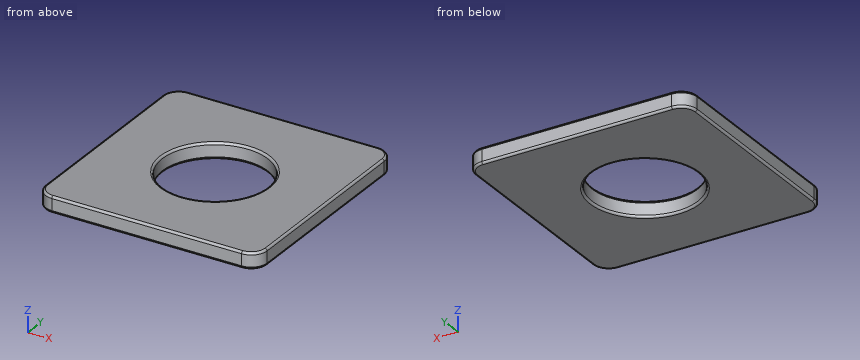
```python
from build123d import *

# Parameters (mm, degrees)
SKETCH1_W           = 21
SKETCH1_H           = 21
BOSS_EXTRUDE1_DEPTH = 0.75
FILLET1_R           = 1.5
SKETCH2_R           = 5
CUT_EXTRUDE1_DEPTH  = 15.924811557
FILLET2_R           = 0.2


with BuildPart() as part:
    # Sketch1 → Boss-Extrude1 (new, symmetric)
    with BuildSketch(Plane.XY):
        Rectangle(SKETCH1_W, SKETCH1_H)
    extrude(amount=BOSS_EXTRUDE1_DEPTH, both=True)

    # Fillet1
    fillet1_edges = [part.edges().sort_by_distance(p)[0] for p in [
        (-10.5, 10.5, 0),
        (10.5, 10.5, 0),
        (10.5, -10.5, 0),
        (-10.5, -10.5, 0),
    ]]
    fillet(fillet1_edges, radius=FILLET1_R)

    # Sketch2 → Cut-Extrude1 (cut, through all)
    with BuildSketch(Plane(origin=(0, 0, -0.75), x_dir=(-1, 0, 0), z_dir=(0, 0, -1))):
        Circle(SKETCH2_R)
    extrude(amount=-CUT_EXTRUDE1_DEPTH, mode=Mode.SUBTRACT)

    # Fillet2
    fillet2_edges = [part.edges().sort_by_distance(p)[0] for p in [
        (-10.5, 0, -0.75),
        (-10.5, 0, 0.75),
        (0, 10.5, -0.75),
        (10.5, 0, -0.75),
        (0, -10.5, -0.75),
        (10.060660172, 10.060660172, -0.75),
        (-10.060660172, -10.060660172, -0.75),
        (10.060660172, -10.060660172, -0.75),
        (-10.060660172, 10.060660172, -0.75),
        (0, 10.5, 0.75),
        (0, -10.5, 0.75),
        (10.5, 0, 0.75),
        (10.060660172, 10.060660172, 0.75),
        (-10.060660172, -10.060660172, 0.75),
        (10.060660172, -10.060660172, 0.75),
        (-10.060660172, 10.060660172, 0.75),
        (5, 0, 0.75),
        (5, 0, -0.75),
    ]]
    fillet(fillet2_edges, radius=FILLET2_R)


solid = part.part
```
The model under review builds one solid part; all positions refer to its coordinate system, in mm. Give positions to 0.01 mm unless a question says otherwise; leave off trailing zeros. Write each loop counter-clockwise with the first axis right and the second up, starting at its lowest first coordinate (ties: lowest second). Pieces come first, ordered by that corner, then holes. Notation, with made-up numbers: M 2,59.25 L 15,59.25 A29 cw 15,91.25 Z; hole C 36,43 d7. An arc over 180 degrees is marked long. Write item = value, one per line. Start each with the question number.
Q1. For line 1 (Y direction, x = 0, z = -0.15); line 2 (Y direction, x = -4, z = -0.05); line 3 (Y direction, x = 8, z = -0.6), list the stretches that pass through material, from the lowest coordinate up.
Q2. Clearance check with flat-ended pins moving along their axes: pin 1 (8 mm diameter, centred on x = -4, y = 0, fed in from +Z); pin 2 (3 mm diameter, centred on x = -3, y = 1, fed in from -Z). State where each tip first meets the part, or that it passes through.
Q3. We need section C-C (z = 0.2). State the section outline as (x, y) points, plus the area to 3 significant figures.
Q4. We need section A-A (y = 0). State the section outline as (x, z) points.
Result set:
q1.line_1 = -10.5 to -5, 5 to 10.5
q1.line_2 = -10.5 to -3, 3 to 10.5
q1.line_3 = -10.49 to 10.49
q2.pin_1 = 0.75
q2.pin_2 = through
q3.outline = M -10.5,-9 A1.5 ccw -9,-10.5 L 9,-10.5 A1.5 ccw 10.5,-9 L 10.5,9 A1.5 ccw 9,10.5 L -9,10.5 A1.5 ccw -10.5,9 Z; hole C 0,0 d10
q3.area = 361 mm2
q4.outline = M -10.5,-0.55 A0.2 ccw -10.3,-0.75 L -5.2,-0.75 A0.2 ccw -5,-0.55 L -5,0.55 A0.2 ccw -5.2,0.75 L -10.3,0.75 A0.2 ccw -10.5,0.55 Z; M 5,-0.55 A0.2 ccw 5.2,-0.75 L 10.3,-0.75 A0.2 ccw 10.5,-0.55 L 10.5,0.55 A0.2 ccw 10.3,0.75 L 5.2,0.75 A0.2 ccw 5,0.55 Z
